Part model, mm, in its own coordinate system. Face numbers are marked on the shaded views. A direction names the side the tool comes from. Give positions to 0.01 mm unless a question says otherwise; leave off trailing zeros. Order: outer loops, then holes, each group sorted by start corner. A loop starts at its lowest first (then second) coordinate and runs counter-clockwise, first axis right, second up. Notation, with made-up numbers: (33, 36) - (51, 36) arc R6 ccw to (51, 47) - close; hole circle Ø8 at (54, -25). An arc over 180 degrees is marked (long way). One line per item, written item: value.
```python
from build123d import *

# Parameters (mm, degrees)
BOSS_EXTRUDE1_DEPTH = 11
SKETCH3_W           = 6.5
SKETCH3_H           = 1.5
CUT_EXTRUDE5_DEPTH  = 3
SKETCH6_R           = 1.5
CUT_EXTRUDE7_DEPTH  = 27.551836095
EXTRUDE_START       = 3
EXTRUDE_1_DEPTH     = 3


with BuildPart() as part:
    # Sketch1 → Boss-Extrude1 (new body)
    with BuildSketch(Plane.XY):
        with BuildLine():
            Line((0.5, 1.5), (0.5, 11.5))
            Line((0.5, 11.5), (15.5, 11.5))
            Line((15.5, 11.5), (15.5, 1.5))
            Line((15.5, 1.5), (22, 1.5))
            Line((22, 1.5), (22, 0))
            Line((22, 0), (14, 0))
            Line((14, 0), (14, 9))
            ThreePointArc((14, 9), (13.707106781, 9.707106781), (13, 10))
            Line((13, 10), (3, 10))
            ThreePointArc((3, 10), (2.292893219, 9.707106781), (2, 9))
            Line((2, 9), (2, 0))
            Line((2, 0), (-6, 0))
            Line((-6, 0), (-6, 1.5))
            Line((-6, 1.5), (0.5, 1.5))
        make_face()
    extrude(amount=BOSS_EXTRUDE1_DEPTH)

    # Sketch3 → Cut-Extrude5 (cut)
    with BuildSketch(Plane.XY.offset(11)):
        with Locations((-2.75, 0.75)):
            Rectangle(SKETCH3_W, SKETCH3_H)
        with Locations((18.75, 0.75)):
            Rectangle(SKETCH3_W, SKETCH3_H)
    extrude(amount=-CUT_EXTRUDE5_DEPTH, mode=Mode.SUBTRACT)

    # Sketch6 → Cut-Extrude7 (cut, through all)
    with BuildSketch(Plane(origin=(0, 1.5, 0), x_dir=(1, 0, 0), z_dir=(0, 1, 0))):
        with Locations(Location((-2.75, -4, 0), (0, 0, 180))):
            Circle(SKETCH6_R)
        with Locations((18.75, -4)):
            Circle(SKETCH6_R)
        Polygon((-6, -1.5), (-4.5, 0), (-6, 0), align=None)
        Polygon((20.5, 0), (22, 0), (22, -1.5), align=None)
        Polygon((22, -6.5), (20.5, -8), (22, -8), align=None)
        Polygon((-4.5, -8), (-6, -8), (-6, -6.5), align=None)
    extrude(amount=-CUT_EXTRUDE7_DEPTH, mode=Mode.SUBTRACT)

    # 草图1 → 凸台-拉伸1 (add)
    with BuildSketch(Plane(origin=(0, 0, 0), x_dir=(-1, 0, 0), z_dir=(0, 0, -1)).offset(EXTRUDE_START)):
        with BuildLine():
            Line((-0.5, 1.5), (-0.5, 0))
            Line((-0.5, 0), (-2, 0))
            Line((-2, 0), (-2, 9))
            ThreePointArc((-2, 9), (-2.292893219, 9.707106781), (-3, 10))
            Line((-3, 10), (-13, 10))
            ThreePointArc((-13, 10), (-13.707106781, 9.707106781), (-14, 9))
            Line((-14, 9), (-14, 0))
            Line((-14, 0), (-15.5, 0))
            Line((-15.5, 0), (-15.5, 1.5))
            Line((-15.5, 1.5), (-15.5, 11.5))
            Line((-15.5, 11.5), (-0.5, 11.5))
            Line((-0.5, 11.5), (-0.5, 1.5))
        make_face()
    extrude(amount=-EXTRUDE_1_DEPTH)


solid = part.part
```
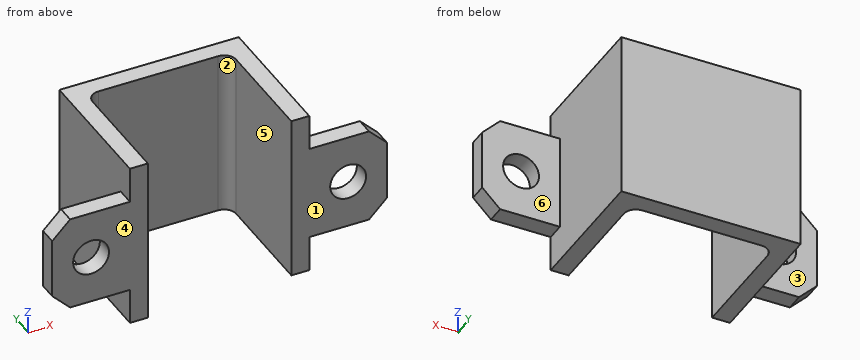
1) Mould opens along X. For the marked faces 1 and 2 say: released by +X, released by -X, zero draft, split by the parting line, or undercut.
Outcome:
face 1: zero draft
face 2: undercut
2) Pin check, flat tips, straight feed: pin 1 (4 mm diameter, centred on y = 9.5, z = 0.5, fed in from +X); pin 2 (3 mm diameter, centred on x = 6.5, z = 0.5, fed in from -Y); pin 3 (2 mm diameter, centred on x = 19.5, z = 4.5, fed in from +Y). Stop position of each tip, or through.
Outcome:
pin 1: stops at x = 15.5
pin 2: stops at y = 10
pin 3: stops at y = 1.5
3) Cut at A-A, the plane x = 18.75. Give the cut face in (y, z), then the cut area to 3 significant figures.
Outcome:
outline: (0, 0) - (1.5, 0) - (1.5, 2.5) - (0, 2.5) - close; (0, 5.5) - (1.5, 5.5) - (1.5, 8) - (0, 8) - close
area: 7.50 mm^2
4) Which spindle directions (+Z, -Z, +X, -X, +Y, -Y) get a long thin tool onto all of the face, cutting with end or side? Do the marked faces 3, 4, 5 and 6. Say none if no direction does.
Outcome:
face 3: +Z, -Z, -X, +Y
face 4: +Z, -Z, +X, -X, -Y
face 5: +Z, -Z, -Y
face 6: +Z, -Z, +X, +Y
5) Cut at D-D, the plane z = 7.5. Give the cut face in (x, y), then the cut area to 3 significant figures.
Outcome:
outline: (-5, 0) - (2, 0) - (2, 9) arc R1 cw to (3, 10) - (13, 10) arc R1 cw to (14, 9) - (14, 0) - (21, 0) - (21, 1.5) - (15.5, 1.5) - (15.5, 11.5) - (0.5, 11.5) - (0.5, 1.5) - (-5, 1.5) - close
area: 69.4 mm^2
6) Cut at B-B, the plane y = 4.25. Give the cut face in (x, z), then the cut area to 3 significant figures.
Outcome:
outline: (0.5, -3) - (2, -3) - (2, 11) - (0.5, 11) - close; (14, -3) - (15.5, -3) - (15.5, 11) - (14, 11) - close
area: 42.0 mm^2
7) Drill centre lines: line 1 along Z through (x, y) = (18.75, 1.1); line 2 along X through (y, z) = (6, 8); line 3 along Y through (x, z) = (11.5, 2.25). Where is each one in solid material? Low to high. Write a range as from..to.
Outcome:
line 1: z = 0..2.5, 5.5..8
line 2: x = 0.5..2, 14..15.5
line 3: y = 10..11.5
8) Cut at C-C, the plane z = 4. Give the cut face in (x, y), then the cut area to 3 significant figures.
Outcome:
outline: (-6, 0) - (-4.25, 0) - (-4.25, 1.5) - (-6, 1.5) - close; (-1.25, 0) - (2, 0) - (2, 9) arc R1 cw to (3, 10) - (13, 10) arc R1 cw to (14, 9) - (14, 0) - (17.25, 0) - (17.25, 1.5) - (15.5, 1.5) - (15.5, 11.5) - (0.5, 11.5) - (0.5, 1.5) - (-1.25, 1.5) - close; (20.25, 0) - (22, 0) - (22, 1.5) - (20.25, 1.5) - close
area: 63.4 mm^2
